```python
from build123d import *

# Parameters (mm, degrees)
ESQUISSE1_W             = 100
ESQUISSE1_H             = 66
BOSS_EXTRU_1_DEPTH      = 40
COQUE1_T                = -3
BOSS_EXTRU_2_DEPTH      = 40
ESQUISSE3_W             = 94
ESQUISSE3_H             = 17
BOSS_EXTRU_3_DEPTH      = 3
CONG_1_R                = 2
CONG_2_R                = 5
BOSS_EXTRU_4_START      = -10
BOSS_EXTRU_4_DEPTH      = 80
BOSS_EXTRU_5_START      = -10
BOSS_EXTRU_5_DEPTH      = 56
ESQUISSE6_W             = 30
ESQUISSE6_H             = 10
ENL_V_MAT_EXTRU_1_DEPTH = 5
ESQUISSE7_R             = 5.05
ESQUISSE7_R_2           = 5
BOSS_EXTRU_6_DEPTH      = 5
ESQUISSE8_R             = 2.05
ENL_V_MAT_EXTRU_2_DEPTH = 81.876448982
BOSS_EXTRU_7_START      = -25.5
BOSS_EXTRU_7_DEPTH      = 25.5
ESQUISSE11_W            = 14
ESQUISSE11_H            = 8
ENL_V_MAT_EXTRU_4_DEPTH = 10
CONG_3_R                = 1
ESQUISSE12_W            = 26
ESQUISSE12_H            = 4
ENL_V_MAT_EXTRU_5_DEPTH = 10


with BuildPart() as part:
    # Esquisse1 → Boss.-Extru.1 (new body)
    with BuildSketch(Plane(origin=(0, 0, 0), x_dir=(1, 0, 0), z_dir=(0, 1, 0))):
        Rectangle(ESQUISSE1_W, ESQUISSE1_H)
    extrude(amount=BOSS_EXTRU_1_DEPTH)

    # Coque1
    coque1_openings = [part.faces().sort_by_distance(p)[0] for p in [
        (0, 40, 0),
    ]]
    offset(amount=COQUE1_T, openings=coque1_openings, kind=Kind.INTERSECTION)

    # Esquisse2 → Boss.-Extru.2 (add)
    with BuildSketch(Plane.XZ):
        Polygon((-50, -33), (-50, -53), (50, -53), (50, -33), (47, -33), (47, -50), (-47, -50), (-47, -33), align=None)
    extrude(amount=-BOSS_EXTRU_2_DEPTH)

    # Esquisse3 → Boss.-Extru.3 (add)
    with BuildSketch(Plane.XZ):
        with Locations((0, -41.5)):
            Rectangle(ESQUISSE3_W, ESQUISSE3_H)
    extrude(amount=-BOSS_EXTRU_3_DEPTH)

    # Congé1
    cong_1_edges = [part.edges().sort_by_distance(p)[0] for p in [
        (47, 21.5, 30),
        (-47, 21.5, 30),
        (-47, 21.5, -50),
        (47, 21.5, -50),
    ]]
    fillet(cong_1_edges, radius=CONG_1_R)

    # Congé2
    cong_2_edges = [part.edges().sort_by_distance(p)[0] for p in [
        (50, 20, -53),
        (-50, 20, -53),
        (50, 20, 33),
        (-50, 20, 33),
    ]]
    fillet(cong_2_edges, radius=CONG_2_R)

    # Esquisse4 → Boss.-Extru.4 (add)
    with BuildSketch(Plane(origin=(50, 0, 0), x_dir=(0, 0, -1), z_dir=(1, 0, 0)).offset(BOSS_EXTRU_4_START)):
        with BuildLine():
            Line((-33, 31), (-33, 29))
            ThreePointArc((-33, 29), (-34, 30), (-33, 31))
        make_face()
    boss_extru_4 = extrude(amount=-BOSS_EXTRU_4_DEPTH)

    # Symétrie1: Boss.-Extru.4 across plane
    add(boss_extru_4.mirror(Plane(origin=(0, 0, -10), x_dir=(1, 0, 0), z_dir=(0, 0, -1))))

    # Esquisse5 → Boss.-Extru.5 (add)
    with BuildSketch(Plane(origin=(0, 0, -53), x_dir=(-1, 0, 0), z_dir=(0, 0, -1)).offset(BOSS_EXTRU_5_START)):
        with BuildLine():
            Line((50, 31), (50, 29))
            ThreePointArc((50, 29), (51, 30), (50, 31))
        make_face()
    boss_extru_5 = extrude(amount=-BOSS_EXTRU_5_DEPTH)

    # Symétrie2: Boss.-Extru.5 across plane
    add(boss_extru_5.mirror(Plane(origin=(0, 0, 0), x_dir=(0, 0, 1), z_dir=(1, 0, 0))))

    # Esquisse6 → Enlèv. mat.-Extru.1 (cut)
    with BuildSketch(Plane.XY.offset(-30)):
        with Locations((-32, 35)):
            Rectangle(ESQUISSE6_W, ESQUISSE6_H)
    extrude(amount=-ENL_V_MAT_EXTRU_1_DEPTH, mode=Mode.SUBTRACT)

    # Esquisse7 → Boss.-Extru.6 (add)
    with BuildSketch(Plane(origin=(0, 3, 0), x_dir=(1, 0, 0), z_dir=(0, 1, 0))):
        with Locations((-33, 25)):
            Circle(ESQUISSE7_R)
        with Locations(Location((-33, -24, 0), (0, 0, 90))):
            Circle(ESQUISSE7_R_2)
        with Locations(Location((39, -18, 0), (0, 0, 90))):
            Circle(ESQUISSE7_R_2)
        with Locations(Location((39, 10, 0), (0, 0, 90))):
            Circle(ESQUISSE7_R_2)
    extrude(amount=BOSS_EXTRU_6_DEPTH)

    # Esquisse8 → Enlèv. mat.-Extru.2 (cut, through all)
    with BuildSketch(Plane(origin=(0, 8, 0), x_dir=(1, 0, 0), z_dir=(0, 1, 0))):
        with Locations(Location((-33, 25, 0), (0, 0, 270))):
            Circle(ESQUISSE8_R)
        with Locations(Location((-33, -24, 0), (0, 0, 270))):
            Circle(ESQUISSE8_R)
        with Locations(Location((39, 10, 0), (0, 0, 270))):
            Circle(ESQUISSE8_R)
        with Locations(Location((39, -18, 0), (0, 0, 270))):
            Circle(ESQUISSE8_R)
    extrude(amount=-ENL_V_MAT_EXTRU_2_DEPTH, mode=Mode.SUBTRACT)

    # Esquisse10 → Boss.-Extru.7 (add)
    with BuildSketch(Plane.XZ.offset(BOSS_EXTRU_7_START)):
        with BuildLine():
            Line((-51.5, 28), (-51.5, -48))
            ThreePointArc((-51.5, -48), (-49.596194078, -52.596194078), (-45, -54.5))
            Line((-45, -54.5), (45, -54.5))
            ThreePointArc((45, -54.5), (49.596194078, -52.596194078), (51.5, -48))
            Line((51.5, -48), (51.5, 28))
            ThreePointArc((51.5, 28), (49.596194078, 32.596194078), (45, 34.5))
            Line((45, 34.5), (-45, 34.5))
            ThreePointArc((-45, 34.5), (-49.596194078, 32.596194078), (-51.5, 28))
        make_face()
        with BuildLine():
            Line((50, 28), (50, -48))
            ThreePointArc((50, -48), (48.535533906, -51.535533906), (45, -53))
            Line((45, -53), (-45, -53))
            ThreePointArc((-45, -53), (-48.535533906, -51.535533906), (-50, -48))
            Line((-50, -48), (-50, 28))
            ThreePointArc((-50, 28), (-48.535533906, 31.535533906), (-45, 33))
            Line((-45, 33), (45, 33))
            ThreePointArc((45, 33), (48.535533906, 31.535533906), (50, 28))
        make_face(mode=Mode.SUBTRACT)
    extrude(amount=BOSS_EXTRU_7_DEPTH)

    # Esquisse11 → Enlèv. mat.-Extru.4 (cut)
    with BuildSketch(Plane(origin=(-47, 0, 0), x_dir=(0, 0, -1), z_dir=(1, 0, 0))):
        with Locations((11.975, 18)):
            Rectangle(ESQUISSE11_W, ESQUISSE11_H)
    extrude(amount=-ENL_V_MAT_EXTRU_4_DEPTH, mode=Mode.SUBTRACT)

    # Congé3
    cong_3_edges = [part.edges().sort_by_distance(p)[0] for p in [
        (-49.25, 22, -18.975),
        (-49.25, 14, -18.975),
        (-49.25, 14, -4.975),
        (-49.25, 22, -4.975),
    ]]
    fillet(cong_3_edges, radius=CONG_3_R)

    # Esquisse12 → Enlèv. mat.-Extru.5 (cut)
    with BuildSketch(Plane(origin=(-47, 0, 0), x_dir=(0, 0, -1), z_dir=(1, 0, 0))):
        with Locations((2.975, 33.5)):
            Rectangle(ESQUISSE12_W, ESQUISSE12_H)
    extrude(amount=-ENL_V_MAT_EXTRU_5_DEPTH, mode=Mode.SUBTRACT)


solid = part.part
```
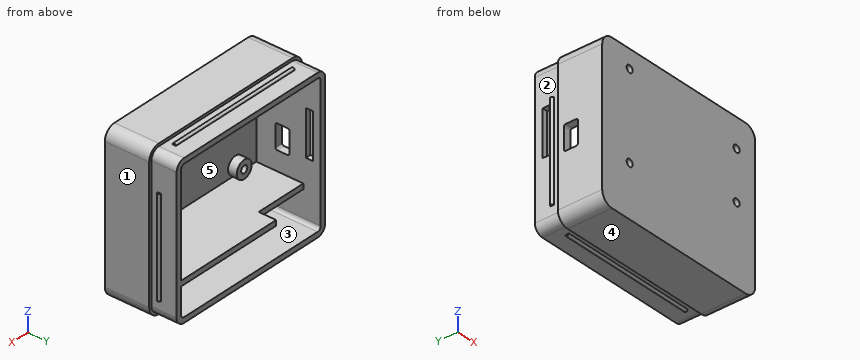
Input: part model. Units: mm. Frame: model coordinates. Face numbers are marked on the shaded views. A direction names the side the tool comes from. Coordinates: 2 decimals unless noted, no trailing zeros. Loops run counter-clockwise (first coordinate to the right, second up) from the corner with the lowest first, then second, coordinate; pieces in that order, holes last. Notation, with made-up numbers: M 48.5,26.5 L 95.5,26.5 A19 cw 95.5,40.5 Z; hole C 30.25,13.5 d9. An arc over 180 degrees is marked long. One line per item, written item: value.
(1) Reachability of the marked faces 4 and 5 from +Z, -Z, +X, -X, +Y, -Y: full face, straight path, thin tool, end or side. Return the list, or none.
Filled in:
face 4: -Z, +X, -X, +Y, -Y
face 5: +Y
(2) Pull-direction query (X, two-part tool) for the marked faces 1, 2 and 3; classes: +X half, -X half, draft (parallel to the pull), parting line (faces both ways), or undercut.
Filled in:
face 1: +X half
face 2: -X half
face 3: undercut
(3) Section C-C (x = 27). Output: boundary loops of the cut face in (y, z), and give its area (3 significant figures).
Filled in:
outline: M 0,-54.5 L 25.5,-54.5 L 25.5,-53 L 29,-53 A1 ccw 31,-53 L 40,-53 L 40,-50 L 3,-50 L 3,-33 L 40,-33 L 40,-30 L 3,-30 L 3,30 L 40,30 L 40,33 L 31,33 A1 ccw 29,33 L 25.5,33 L 25.5,34.5 L 0,34.5 Z
area: 671 mm^2
(4) Pin query (flat end, axial travel): pin 1 (3 mm diameter, centred on x = 7.5, z = 13, fed in from +Y); pin 2 (3.5 mm diameter, centred on x = -48.5, y = 33.5, fed in from +Z); pin 3 (2 mm diameter, centred on x = -31.5, z = 21, fed in from +Y). Return the tip coordinate at first contact, or that it passes through.
Filled in:
pin 1: y = 3
pin 2: z = 32.68
pin 3: y = 8
(5) Section A-A (z = 6). Output: boundary loops of the cut face in (x, y), and give its area (3 significant figures).
Filled in:
outline: M -51.5,0 L 51.5,0 L 51.5,25.5 L 50,25.5 L 50,29 A1 ccw 50,31 L 50,40 L 47,40 L 47,3 L -47,3 L -47,31.5 L -50,31.5 L -50,31 A1 ccw -50,29 L -50,25.5 L -51.5,25.5 Z; M -50,35.5 L -47,35.5 L -47,40 L -50,40 Z
area: 590 mm^2
(6) Section D-D (z = -10). Give the number of separate pieces and of enclosed holes in the cut face, and give its area (3 significant figures).
Filled in:
separate pieces: 4
enclosed holes: 0
area: 571 mm^2
(7) Section B-B (y = 12.5). Output: boundary loops of the cut face in (x, z), and give its area (3 significant figures).
Filled in:
outline: M -51.5,-48 A6.5 ccw -45,-54.5 L 45,-54.5 A6.5 ccw 51.5,-48 L 51.5,28 A6.5 ccw 45,34.5 L -45,34.5 A6.5 ccw -51.5,28 Z; hole M -47,-48 A2 ccw -45,-50 L 45,-50 A2 ccw 47,-48 L 47,-33 L -47,-33 Z; hole M -47,-30 L 47,-30 L 47,28 A2 ccw 45,30 L -45,30 A2 ccw -47,28 Z
area: 1,900 mm^2
(8) Line query: line 1 along X through (y, z) = (4.5, -10); line 2 along Z through (x, y) = (18, 15); line 3 along X through (y, z) = (13, 24). Output: solid intervals per line, ascending. Write a range as from..to.
Filled in:
line 1: -51.5..-47, 34..36.95, 41.05..44, 47..51.5
line 2: -54.5..-50, -33..-30, 30..34.5
line 3: -51.5..-47, 47..51.5
